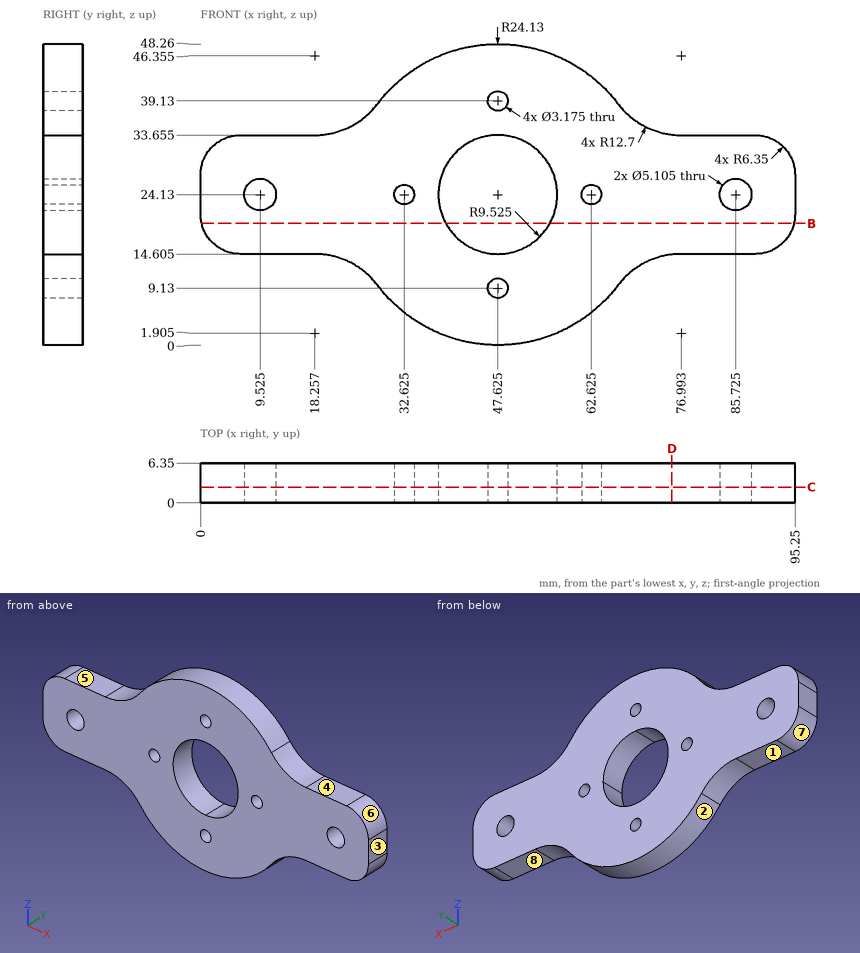
For this review, use the dimensioned drawing (mm, ordinates from the lowest corner) and the shaded views. A direction names the side the tool comes from. Coordinates: 2 decimals unless noted, no trailing zeros. Write each loop counter-clockwise with the first axis right and the second up, starting at its lowest first coordinate (ties: lowest second). Pieces come first, ordered by that corner, then holes. Notation, with made-up numbers: (50.25, 47.5) - (109.25, 47.5) arc R31 ccw to (109.25, 71.5) - close; hole circle Ø11 at (48.25, 40.5). An arc over 180 degrees is marked (long way). Answer as a JSON object with one key per item and string values. Group by question number.
1. To check wall thickness, follow probe 1 along X at (y, z) = (0.5, 24.5); probe 2 along X at (y, z) = (5.25, 38); probe 3 along Z at (x, y) = (56, 5.5) (1 decimal). State the ranges of each line that lie inside material, in increasing order.
2. Add section D-D (x = 75.5). Give the boundary of the cut face in (y, z).
3. Add section C-C (y = 2.5). Give the number of separate pieces and of enclosed holes in the cut face, plus the area to 3 significant figures.
4. Machinability: for the marked faces 1, 2, 3, 4 and 5, which of the approach directions +Z, -Z, +X, -X, +Y, -Y give a long, thin tool a straight path to every point of the face, cutting with its end or side? Answer none if there is none.
5. Mouldability with a two-part tool opening along X and no side actions: class the marked faces 6, 7 and 8 as pulls with the +X half, pulls with the -X half, needs draft (parallel to the pull), parting line crosses it, or undercut.
6. Clearance check with flat-ended pins moving along their axes: pin 1 Ø1.9 at (x, y) = (83, 3.5) entering from -Z (3 decimals); pin 2 Ø3 at (y, z) = (1.5, 14) entering from +X; pin 3 Ø8 at (x, z) = (85.725, 24.13) entering from +Y; pin 4 Ø3 at (y, z) = (5.5, 34.5) entering from -X. State where each tip first meets the part, or that it passes through.
7. Add section B-B (z = 19.5). Give the boundary of the cut face in (x, y).
Findings:
{
 "1": {"probe 1": "0 to 7, 12.05 to 31.08, 34.17 to 38.11, 57.14 to 61.08, 64.17 to 83.2, 88.25 to 95.25", "probe 2": "27.82 to 46.51, 48.74 to 67.43", "probe 3": "1.5 to 19.6, 28.7 to 46.8"},
 "2": {"outline": "(0, 14.52) - (6.35, 14.52) - (6.35, 33.74) - (0, 33.74) - close"},
 "3": {"separate pieces": "1", "enclosed holes": "7", "area": "2,390 mm²"},
 "4": {"face 1": "-Z, -X, +Y, -Y", "face 2": "-Z, +Y, -Y", "face 3": "+Z, -Z, +X, +Y, -Y", "face 4": "+Z, +X, +Y, -Y", "face 5": "+Z, -X, +Y, -Y"},
 "5": {"face 6": "pulls with the +X half", "face 7": "pulls with the -X half", "face 8": "needs draft"},
 "6": {"pin 1": "z = 14.605", "pin 2": "x = 92.15", "pin 3": "y = 6.35", "pin 4": "x = 3.54"},
 "7": {"outline": "(0.17, 0) - (39.3, 0) - (39.3, 6.35) - (0.17, 6.35) - close; (55.95, 0) - (95.08, 0) - (95.08, 6.35) - (55.95, 6.35) - close"}
}
